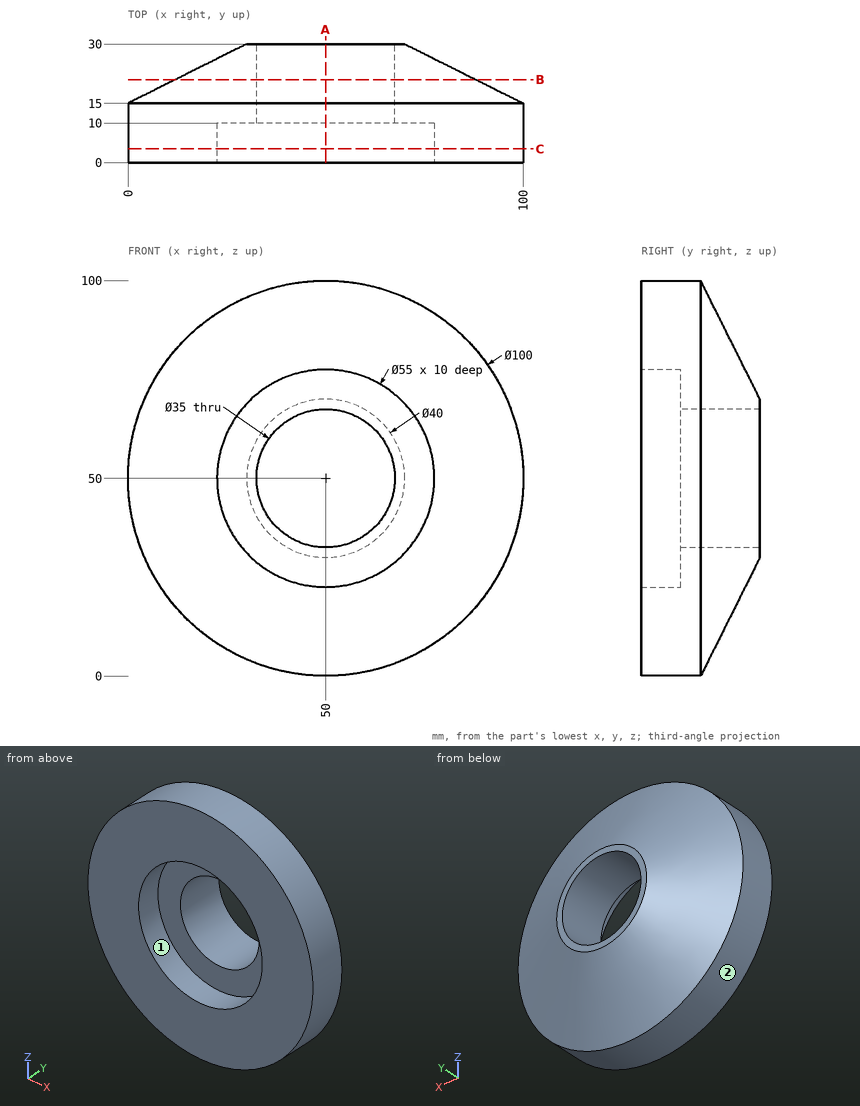
The figure shows three views and two pictorial views of one solid part (mm, origin at its lowest corner). Answer the questions. A direction names the side the tool comes from. Round coordinates to 2 decimals unless told otherwise and drop trailing zeros. Write each loop counter-clockwise with the first axis right and the second up, starting at its lowest first coordinate (ties: lowest second). Pieces come first, ordered by that corner, then holes. Notation, with made-up numbers: M 59,13 L 72,13 A23 cw 72,38 Z; hole C 52.25,64 d1. An arc over 180 degrees is marked long. Use a Markdown table: item, result.
1) The part is cut by section A-A (x = 50). Write down the section's boundary in (y, z).
Answers follow:
| item | result |
|---|---|
| outline | M 0,0 L 15,0 L 30,30 L 30,32.5 L 10,32.5 L 10,22.5 L 0,22.5 Z; M 0,77.5 L 10,77.5 L 10,67.5 L 30,67.5 L 30,70 L 15,100 L 0,100 Z |
2) The part is cut by section C-C (y = 3.5). Write down the section's boundary in (x, z), plus the area to 3 significant figures.
Answers follow:
| item | result |
|---|---|
| outline | C 50,50 d100; hole C 50,50 d55 |
| area | 5,480 mm2 |
3) Straight lines are drawn through the part: line 1 along X through (y, z) = (5, 50); line 2 along X through (y, z) = (5, 28.5); line 3 along Z through (x, y) = (34, 9.5). For each, find the intervals that lie inside material, in ascending order. Write a range as [from, to].
Answers follow:
| item | result |
|---|---|
| line 1 | x = [0, 22.5], [77.5, 100] |
| line 2 | x = [4.86, 32.85], [67.15, 95.14] |
| line 3 | z = [2.63, 27.63], [72.37, 97.37] |
4) The part is cut by section B-B (y = 21). Write down the section's boundary in (x, z).
Answers follow:
| item | result |
|---|---|
| outline | C 50,50 d76; hole C 50,50 d35 |
5) Flat-ended cylindrical pins translate along their axes: pin 1 (1 mm diameter, centred on x = 55, z = 74.5, fed in from -Y); pin 2 (6 mm diameter, centred on x = 57.5, y = 10.5, fed in from +Z); pin 3 (5 mm diameter, centred on y = 14.5, z = 67, fed in from -X). Find the tip coordinate at first contact, or state that the pin passes through.
Answers follow:
| item | result |
|---|---|
| pin 1 | stops at y = 10 |
| pin 2 | stops at z = 99.8 |
| pin 3 | stops at x = 2.15 |
6) A tool of negligible diameter and unlimited length cuts with its end or side. For the marked faces 1 and 2, from which of +Z, -Z, +X, -X, +Y, -Y can it reach the whole face along a straight path? Write none if from no direction.
Answers follow:
| item | result |
|---|---|
| face 1 | -Y |
| face 2 | +Y, -Y |
